Geometry: final body of the model. Coordinates: model frame, mm. A direction names the side the tool comes from. Give positions to 0.01 mm unless a question says otherwise; leave off trailing zeros. Write each loop counter-clockwise with the first axis right and the second up, starting at its lowest first coordinate (ties: lowest second). Pieces come first, ordered by that corner, then holes. Notation, with made-up numbers: (-6.75, 86.5) -> (6.25, 86.5) arc R17 ccw to (6.25, 118.5) -> close; hole circle Ø5 at (0.25, -17.5). An arc over 180 degrees is marked (long way). Answer in a Markdown table with one row per item. Add a question column.
Item 1: Section query B-B on z = 9. Output: boundary loops of the cut face in (x, y), plus the area to 3 significant figures.
Item 2: Section query A-A on x = 0. Output: boundary loops of the cut face in (y, z), plus the area to 4 significant figures.
Item 3: Section query C-C on y = 0. Output: boundary loops of the cut face in (x, z), plus the area to 3 significant figures.
Item 4: Draft query along X for faces 4 (the conical face through (6.7, -0.1, 0.2)), 5 (the flat face through (4, 0, 0)), 6 (the flat face through (-4, 0, 4)). Return one class per face: +X half, -X half, draft (parallel to the pull), parting line (faces both ways), or undercut.
Item 5: First-contact query: P1, Ø5, axis at x = -3, z = 20, coming from the +Y side; P2, Ø3, axis at y = -2, z = 7, coming from the -X side; P3, Ø3, axis at x = 0.5, y = 1.5, coming from the -Z side. Flat tips, straight axial feed; report the tip coordinate or a pass-through.
Item 6: Access query for faces 1 (the flat face through (-3.1, 0, 2)), 2 (the cylindrical face through (-7.493, 0.33, 11.846)), 3 (the flat face through (4, 0, 4)). Directions: +Z, -Z, +X, -X, +Y, -Y. A direction counts if a zero-diameter tool reaches every point of the face in a straight line with its end or side. Return the directions, or none.
Item 7: Material intervals for probe 1 along X at (y, z) = (-0.25, 8.75); probe 2 along Z at (x, y) = (-3, 3.25); probe 3 along X at (y, z) = (4, 5.25), sorted ascending. Write a range as from..to.
Item 8: Section query D-D on z = 17. Output: boundary loops of the cut face in (x, y), plus the area to 3 significant figures.
```python
from build123d import *

# Parameters (mm, degrees)
SKETCH_1_R          = 7.5
EXTRUDE_1_DEPTH     = 24
CUT_EXTRUDE_1_DEPTH = 10
CHAMFER_1_SIZE      = 1
CHAMFER_2_SIZE      = 1


with BuildPart() as part:
    # 草图1 → 凸台-拉伸1 (new body)
    with BuildSketch(Plane.XY):
        Circle(SKETCH_1_R)
    extrude(amount=EXTRUDE_1_DEPTH)

    # 草图2 → 切除-拉伸1 (cut, symmetric)
    with BuildSketch(Plane(origin=(0, 0, 0), x_dir=(1, 0, 0), z_dir=(0, 1, 0))):
        Polygon((3.1, 0), (-3.1, 0), (-3.1, -4), (-5.1, -4), (-5.1, -10.1), (5.1, -10.1), (5.1, -4), (3.1, -4), align=None)
    extrude(amount=CUT_EXTRUDE_1_DEPTH, both=True, mode=Mode.SUBTRACT)

    # 倒角1
    chamfer_1_edges = [part.edges().sort_by_distance(p)[0] for p in [
        (-7.5, 0, 24),
    ]]
    chamfer(chamfer_1_edges, length=CHAMFER_1_SIZE)

    # 倒角2
    chamfer_2_edges = [part.edges().sort_by_distance(p)[0] for p in [
        (-7.5, 0, 0),
        (6.304760106, -4.062019202, 0),
    ]]
    chamfer(chamfer_2_edges, length=CHAMFER_2_SIZE)


solid = part.part
```
Findings below:
| question | item | result |
|---|---|---|
| 1 | outline | (-5.1, -5.5) -> (-5.1, 5.5) arc R7.5 ccw to start; (5.1, -5.5) arc R7.5 ccw to (5.1, 5.5) -> close |
| 1 | area | 36.5 mm^2 |
| 2 | outline | (-7.5, 10.1) -> (7.5, 10.1) -> (7.5, 23) -> (6.5, 24) -> (-6.5, 24) -> (-7.5, 23) -> close |
| 2 | area | 207.5 mm^2 |
| 3 | outline | (-7.5, 1) -> (-6.5, 0) -> (-3.1, 0) -> (-3.1, 4) -> (-5.1, 4) -> (-5.1, 10.1) -> (5.1, 10.1) -> (5.1, 4) -> (3.1, 4) -> (3.1, 0) -> (6.5, 0) -> (7.5, 1) -> (7.5, 23) -> (6.5, 24) -> (-6.5, 24) -> (-7.5, 23) -> close |
| 3 | area | 271 mm^2 |
| 4 | face 4 | +X half |
| 4 | face 5 | draft |
| 4 | face 6 | undercut |
| 5 | P1 | stops at y = 7.48 |
| 5 | P2 | stops at x = -7.48 |
| 5 | P3 | stops at z = 10.1 |
| 6 | face 1 | -Z, +Y, -Y |
| 6 | face 2 | +Z, -Z |
| 6 | face 3 | +Y, -Y |
| 7 | probe 1 | x = -7.5..-5.1, 5.1..7.5 |
| 7 | probe 2 | z = 10.1..24 |
| 7 | probe 3 | x = -6.34..-5.1, 5.1..6.34 |
| 8 | outline | circle Ø15 at (0, 0) |
| 8 | area | 177 mm^2 |
